Model file for the job. Use its own axes, mm. A direction names the side the tool comes from. Coordinates: 2 decimals unless noted, no trailing zeros. Write each loop counter-clockwise with the first axis right and the second up, starting at its lowest first coordinate (ties: lowest second). Pieces come first, ordered by that corner, then holes.
Q1. Band-saw the part on C-C, the plane x = 11.5. Write the cut outline in (y, z), plus the area to 3 significant figures.
Q2. Band-saw the part on A-A, the plane y = -62.5. Write the cut outline in (x, z).
Q3. Band-saw the part on B-B, the plane y = -17.5. Write the cut outline in (x, z), plus the area to 3 significant figures.
Q4. Drill centre lines: probe 1 along Y at (x, z) = (-86, 1); probe 2 along Y at (x, z) = (-56.5, 0.4); probe 3 along X at (y, z) = (-99, 1.5). Where is each one in solid material? Low to high.
Q5. Pin check, flat tips, straight feed: P1, Ø12, axis at x = -74.5, y = -27.5, coming from the -Z side; P2, Ø0.6, axis at x = 77.5, z = 0.5, coming from the +Y side; P3, Ø0.6, axis at x = -90, z = 1, coming from the +Y side; P4, Ø0.8, axis at y = 23, z = 1, coming from the -X side. Stop position of each tip, or through.
Q6. Band-saw the part on D-D, the plane x = -41. Write the cut outline in (y, z).
Q7. Which spindle directions (+Z, -Z, +X, -X, +Y, -Y) get a long thin tool onto all of the face, cutting with end or side? Do faces 5 (the flat face through (-1.112, 18.148, 0.986)), 6 (the flat face through (-11, 28, 2)). Say none if no direction does.
Q8. Pull direction X, two halves, no side cores. Call faces 1 (the flat face through (-67.745, -54.522, 0.986)), 2 (the flat face through (-11, 28, 0)), 3 (the flat face through (-88.3, 47.02, 0.99)), 4 (the flat face through (10.15, 46.81, 0.99)): released by +X, released by -X, zero draft, split by the parting line, or undercut.
from build123d import *

# Parameters (mm, degrees)
EXTRUDE_1_DEPTH = 2
FILLET_1_R      = 2


with BuildPart() as part:
    # 草图1 → 凸台-拉伸1 (new body)
    with BuildSketch(Plane.XY):
        Polygon((81.606020908, 1.417469639), (81.606020908, 9.417469639), (76.606020908, 9.417469639), (76.606020908, 18.417469797), (72.606020908, 18.417469797), (72.606020908, 16.917469797), (69.406020908, 16.917469797), (69.406020908, 18.417469797), (66.206020908, 18.417469797), (66.206020908, 22.417469797), (69.406020908, 22.417469797), (69.406020908, 23.917469797), (72.606020908, 23.917469797), (72.606020908, 22.417469797), (76.606020908, 22.417469797), (76.606020908, 31.417469956), (81.606020908, 31.417469956), (81.606020908, 39.417469956), (76.606020908, 39.417469956), (49.568659109, 39.417469956), (-30.393979092, 54.417469639), (-81.393979092, 54.417469639), (-95.393979092, 39.417469956), (-100.393979092, 39.417469956), (-100.393979092, 31.417469956), (-95.393979092, 31.417469956), (-95.393979092, 22.417469797), (-91.393979092, 22.417469797), (-91.393979092, 23.917469797), (-88.193979092, 23.917469797), (-88.193979092, 22.417469797), (-84.993979092, 22.417469797), (-84.993979092, 18.417469797), (-88.193979092, 18.417469797), (-88.193979092, 16.917469797), (-91.393979092, 16.917469797), (-91.393979092, 18.417469797), (-95.393979092, 18.417469797), (-95.393979092, 9.417469639), (-100.393979092, 9.417469639), (-100.393979092, 1.417469639), (-95.393979092, 1.417469639), (-95.393979092, -72.582530044), (-100.393979092, -72.582530044), (-100.393979092, -80.582530044), (-95.393979092, -80.582530044), (-95.393979092, -89.582530203), (-91.393979092, -89.582530203), (-91.393979092, -88.082530203), (-88.193979092, -88.082530203), (-88.193979092, -89.582530203), (-84.993979092, -89.582530203), (-84.993979092, -93.582530203), (-88.193979092, -93.582530203), (-88.193979092, -95.082530203), (-91.393979092, -95.082530203), (-91.393979092, -93.582530203), (-95.393979092, -93.582530203), (-95.393979092, -102.582530361), (-100.393979092, -102.582530361), (-100.393979092, -110.582530361), (-95.393979092, -110.582530361), (-74.110124615, -110.582530361), (-61.393979092, 1.417469639), (-61.393979092, 34.417469639), (-50.393979092, 34.417469639), (49.568659109, 1.417469639), (55.241335591, -110.582530361), (76.606020908, -110.582530361), (81.606020908, -110.582530361), (81.606020908, -102.582530361), (76.606020908, -102.582530361), (76.606020908, -93.582530203), (72.606020908, -93.582530203), (72.606020908, -95.082530203), (69.406020908, -95.082530203), (69.406020908, -93.582530203), (66.206020908, -93.582530203), (66.206020908, -89.582530203), (69.406020908, -89.582530203), (69.406020908, -88.082530203), (72.606020908, -88.082530203), (72.606020908, -89.582530203), (76.606020908, -89.582530203), (76.606020908, -80.582530044), (81.606020908, -80.582530044), (81.606020908, -72.582530044), (76.606020908, -72.582530044), (76.606020908, 1.417469639), align=None)
    extrude(amount=EXTRUDE_1_DEPTH)

    # 圆角1
    fillet_1_edges = [part.edges().sort_by_distance(p)[0] for p in [
        (81.606020908, -102.582530361, 1),
        (81.606020908, -110.582530361, 1),
        (55.241335591, -110.582530361, 1),
        (-61.393979092, 34.417469639, 1),
        (-61.393979092, 1.417469639, 1),
        (-74.110124615, -110.582530361, 1),
        (-100.393979092, -110.582530361, 1),
        (-100.393979092, -102.582530361, 1),
        (-100.393979092, -80.582530044, 1),
        (-100.393979092, -72.582530044, 1),
        (-100.393979092, 1.417469639, 1),
        (-100.393979092, 9.417469639, 1),
        (-100.393979092, 31.417469956, 1),
        (-100.393979092, 39.417469956, 1),
        (81.606020908, 31.417469956, 1),
        (81.606020908, 9.417469639, 1),
        (81.606020908, 1.417469639, 1),
        (81.606020908, -72.582530044, 1),
        (81.606020908, -80.582530044, 1),
    ]]
    fillet(fillet_1_edges, radius=FILLET_1_R)


solid = part.part
Answer sheet:
1. outline: (13.98, 0) - (46.56, 0) - (46.56, 2) - (13.98, 2) - close
1. area: 65.1 mm2
2. outline: (-95.39, 0) - (-68.65, 0) - (-68.65, 2) - (-95.39, 2) - close; (52.81, 0) - (76.61, 0) - (76.61, 2) - (52.81, 2) - close
3. outline: (-95.39, 0) - (-63.54, 0) - (-63.54, 2) - (-95.39, 2) - close; (50.53, 0) - (76.61, 0) - (76.61, 2) - (50.53, 2) - close
3. area: 116 mm2
4. probe 1: y = -110.58 to -93.58, -89.58 to 18.42, 22.42 to 49.48
4. probe 2: y = 34.42 to 54.42
4. probe 3: x = -95.39 to -72.8, 54.65 to 76.61
5. P1: stops at z = 0
5. P2: stops at y = 39.42
5. P3: stops at y = 45.52
5. P4: stops at x = -95.39
6. outline: (31.32, 0) - (54.42, 0) - (54.42, 2) - (31.32, 2) - close
7. face 5: +Z, -Z, -Y
7. face 6: +Z, +X, -X, +Y, -Y
8. face 1: undercut
8. face 2: zero draft
8. face 3: released by -X
8. face 4: released by +X
